from build123d import *

# Parameters (mm, degrees)
F0_W     = 100
F0_H     = 100
F1_DEPTH = 100
F2_W     = 100
F2_H     = 93.59855
F3_DEPTH = 50
F4_W     = 84.22891
F4_H     = 40.867575
F5_DEPTH = 75
F6_W     = 65.648086
F6_H     = 30.288235
F7_DEPTH = 25


with BuildPart() as f1:
    # F0 (on Top) → F1 (new body)
    with BuildSketch(Plane.XY):
        Rectangle(F0_W, F0_H)
    extrude(amount=F1_DEPTH)

    # F2 (on face) → F3 (cut)
    with BuildSketch(Plane.XY.offset(100)):
        with Locations((0, -3.200725)):
            Rectangle(F2_W, F2_H)
    extrude(amount=-F3_DEPTH, mode=Mode.SUBTRACT)

    # F4 (on face) → F5 (cut)
    with BuildSketch(Plane.XZ.offset(50)):
        with Locations((0, 20.151093)):
            Rectangle(F4_W, F4_H)
    extrude(amount=-F5_DEPTH, mode=Mode.SUBTRACT)

    # F6 (on face) → F7 (cut)
    with BuildSketch(Plane.YZ.offset(50)):
        with Locations((0, 24.784692)):
            Rectangle(F6_W, F6_H)
    extrude(amount=-F7_DEPTH, mode=Mode.SUBTRACT)


solid = f1.part
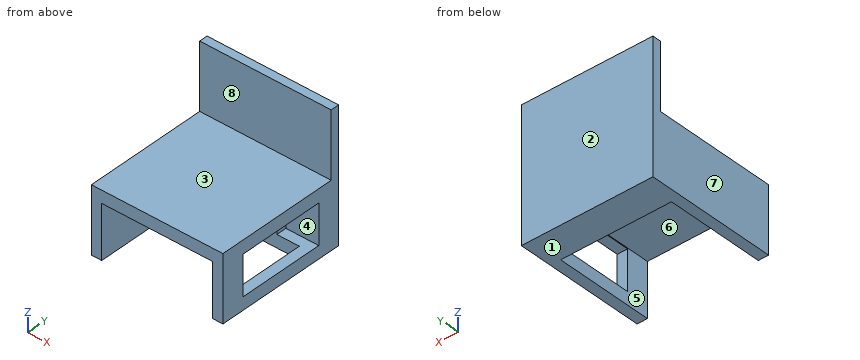
The listing builds one solid part. Answer for the finished solid, in the listing's coordinates (mm). Face numbers are marked on the shaded views. A direction names the side the tool comes from. Coordinates: 2 decimals unless noted, no trailing zeros. Write each loop counter-clockwise with the first axis right and the second up, starting at its lowest first coordinate (ties: lowest second). Pieces come first, ordered by that corner, then holes. Notation, with made-up numbers: M -17,82 L -13,82 A22 ccw -13,93 Z; hole C 41.25,48 d3. An arc over 180 degrees is marked long. Put each result on its own line as item: value. Start each with the question number.
1. For a pull along X with two mould halves and no side action, classify the marked faces 6, 7 and 8 as pulls with the +X half, pulls with the -X half, needs draft (parallel to the pull), parting line crosses it, or undercut.
2. A cutting plane is placed at A-A on y = 21. Write down the section's boundary in (x, z), then the cut area to 3 significant figures.
3. Consider line 1 (Y direction, x = 43.5, z = 28); line 2 (X direction, y = -39.5, z = 24.5); line 3 (Y direction, x = 39, z = 59). Determine where each line is inside the solid, lowest interval first. Write a range as from..to.
4. A cutting plane is placed at D-D on x = -5. Write down the section's boundary in (y, z).
5. A cutting plane is placed at B-B on z = 14. Write down the section's boundary in (x, y).
6. A cutting plane is placed at C-C on y = -38.5. Write down the section's boundary in (x, z), then the cut area to 3 significant figures.
7. Which of the six approach directions +Z, -Z, +X, -X, +Y, -Y give full straight-line access (tool end or side, diameter ignored) to the marked faces 1, 2, 3, 4 and 5?
8. Flat-ended cylindrical pins translate along their axes: P1, Ø4, axis at x = 13.5, y = -24, coming from the +Z side; P2, Ø20, axis at x = 31.5, y = 4, coming from the -Z side; P3, Ø5, axis at x = 12, z = 19.5, coming from the -Y side; P4, Ø6, axis at y = -0.5, z = 53.5, coming from the +X side. Find the tip coordinate at first contact, or state that the pin passes through.
Resolved:
1. face 6: undercut
1. face 7: pulls with the -X half
1. face 8: needs draft
2. outline: M -50,0 L -42.11,0 L -42.11,40.58 L 42.11,40.58 L 42.11,39.93 L 50,39.93 L 50,50 L -50,50 Z; M 42.11,0 L 50,0 L 50,9.64 L 42.11,9.64 Z
2. area: 1,340 mm2
3. line 1: y = -50..-32.82, 32.82..50
3. line 2: x = -50..-42.11, 42.11..50
3. line 3: y = 43.6..50
4. outline: M -50,40.58 L 25,40.58 L 25,0 L 50,0 L 50,100 L 43.6,100 L 43.6,50 L -50,50 Z
5. outline: M -50,-50 L -42.11,-50 L -42.11,25 L 25,25 L 25,32.82 L 50,32.82 L 50,50 L -50,50 Z; M 42.11,-50 L 50,-50 L 50,-32.82 L 42.11,-32.82 Z
6. outline: M -50,0 L -42.11,0 L -42.11,40.58 L 42.11,40.58 L 42.11,0 L 50,0 L 50,50 L -50,50 Z
6. area: 1,580 mm2
7. face 1: -Z, +X, -X, +Y, -Y
7. face 2: +Z, -Z, +X, -X, +Y
7. face 3: +Z, +X, -X, -Y
7. face 4: +X
7. face 5: -Z, -Y
8. P1: stops at z = 50
8. P2: stops at z = 40.58
8. P3: stops at y = 25
8. P4: passes through
